from build123d import *

# Parameters (mm, degrees)
BOSS_EXTRUDE1_DEPTH = 30
SKETCH3_R           = 2
CUT_EXTRUDE2_DEPTH  = 29.4
SKETCH11_R          = 10.983403138
CUT_EXTRUDE3_DEPTH  = 80


with BuildPart() as part:
    # Sketch1 → Boss-Extrude1 (new body)
    with BuildSketch(Plane.XY):
        Polygon((14.2, 13.761910466), (-14.2, 13.761910466), (-14.2, 2.5), (-11.082842712, 2.5), (-8, 2.5), (-8, 4.817157288), (-10.782842712, 7.6), (-6.482842712, 11.9), (6.482842712, 11.9), (10.782842712, 7.6), (8, 4.817157288), (8, 2.5), (11.082842712, 2.5), (14.2, 2.5), align=None)
    extrude(amount=BOSS_EXTRUDE1_DEPTH)

    # Sketch3 → Cut-Extrude2 (cut, through all)
    with BuildSketch(Plane(origin=(14.2, 0, 0), x_dir=(0, 0, -1), z_dir=(1, 0, 0))):
        with Locations(Location((-15, 9.5, 0), (0, 0, 90))):  # turned: the seam where the file's is
            Circle(SKETCH3_R)
    extrude(amount=-CUT_EXTRUDE2_DEPTH, mode=Mode.SUBTRACT)

    # Sketch9 → Revolve2 (revolve)
    with BuildSketch(Plane(origin=(0, 0, 0), x_dir=(0, 0, -1), z_dir=(1, 0, 0))):
        with BuildLine():
            Line((-28.483403138, 93.761910466), (-15, 93.761910466))
            Line((-15, 93.761910466), (-15, 13.761910466))
            Line((-15, 13.761910466), (-28.483403138, 13.761910466))
            add(Edge.make_bspline(
                [(-28.483403138, 13.761910466), (-31.145086737, 24.692296315), (-27.121377906, 28.762236937), (-30.913064787, 43.557319505), (-27.295577593, 49.132991937), (-31.19480755, 65.565333342), (-25.775389052, 74.245854005), (-31.645928371, 82.017446749), (-28.483403138, 93.761910466)],
                knots=[0, 0, 0, 0, 0.086706603, 0.114658805, 0.26120389, 0.315545924, 0.639761013, 1, 1, 1, 1], degree=3))
        make_face()
    revolve(axis=Axis((0, 13.761910466, 15), (0, 1, 0)))

    # Sketch11 → Cut-Extrude3 (cut)
    with BuildSketch(Plane(origin=(0, 93.761910466, 0), x_dir=(1, 0, 0), z_dir=(0, 1, 0))):
        with Locations(Location((0, -15, 0), (0, 0, 270))):  # turned: the seam where the file's is
            Circle(SKETCH11_R)
    extrude(amount=-CUT_EXTRUDE3_DEPTH, mode=Mode.SUBTRACT)


solid = part.part
The model under review builds one solid part; all positions refer to its coordinate system, in mm. A direction names the side the tool comes from. Coordinates: 2 decimals unless noted, no trailing zeros. Loops run counter-clockwise (first coordinate to the right, second up) from the corner with the lowest first, then second, coordinate; pieces in that order, holes last. Notation, with made-up numbers: M 24.5,-12.75 L 41.5,-12.75 A11 cw 41.5,-4.75 Z; hole C 53,-30.5 d10. An arc over 180 degrees is marked long. Put each result on its own line as item: value. Start each with the question number.
Q1. Wall thickness on line 1 (Y direction, x = -6.25, z = 4); line 2 (Y direction, x = -4.25, z = 9.5); line 3 (X direction, y = 42, z = 18): over which ranges is each line inside the solid? List them lowest first.
Q2. The part is to be moulded in two halves that separate along Y. For faces 6 (the cylindrical face through (-11.303, 11.408, 15.601)), 7 (the flat face through (6.692, 11.691, 14.79)), 8 (the flat face through (0, 13.762, 15)), 9 (the flat face through (0, 13, 0)), say which applies: +Y half, -Y half, draft (parallel to the pull), parting line (faces both ways), or undercut.
Q3. Clearance check with flat-ended pins moving along their axes: pin 1 (10.5 mm diameter, centred on x = -1, z = 11.5, fed in from -Y); pin 2 (12.5 mm diameter, centred on y = 10, z = 10, fed in from +X); pin 3 (1 mm diameter, centred on x = -3, z = 13.5, fed in from +Y). State where each tip first meets the part, or that it passes through.
Q4. Add section A-A (y = 9.5). Write out the cut boundary in (x, z), and give its area (3 significant figures).
Q5. For faces 1 (the flat face through (-14.2, 7, 15)), 2 (the flat face through (-9.372, 6.189, 14.79)), 3 (the flat face through (-8, 4, 15)), 4 (the flat face through (14.2, 7, 15)), 5 (the flat face through (3.2, 13.762, 1.6)), list the 3-axis set-ups (+Z, -Z, +X, -X, +Y, -Y) from which the entire face can be reached by the end or side of a thin tool; tool diameter is ignored.
Answers:
1. line 1: y = 11.9 to 93.76
1. line 2: y = 11.9 to 13.76
1. line 3: x = -14.2 to -10.57, 10.57 to 14.2
2. face 6: undercut
2. face 7: undercut
2. face 8: +Y half
2. face 9: draft
3. pin 1: stops at y = 11.9
3. pin 2: stops at x = 14.2
3. pin 3: stops at y = 13.76
4. outline: M -14.2,0 L -8.88,0 L -8.88,13 L -14.2,13 Z; M -14.2,17 L -8.88,17 L -8.88,30 L -14.2,30 Z; M 8.88,0 L 14.2,0 L 14.2,13 L 8.88,13 Z; M 8.88,17 L 14.2,17 L 14.2,30 L 8.88,30 Z
4. area: 276 mm^2
5. face 1: +Z, -Z, -X, -Y
5. face 2: +Z, -Z
5. face 3: +Z, -Z, -Y
5. face 4: +Z, -Z, +X, -Y
5. face 5: none
